Source: CAD feature listing. Evaluate the final solid. Frame: model axes, mm. Give positions to 0.01 mm unless a question says otherwise; leave off trailing zeros. Write each loop counter-clockwise with the first axis right and the second up, starting at its lowest first coordinate (ties: lowest second). Pieces come first, ordered by that corner, then holes. Notation, with made-up numbers: (14, -32.5) -> (38, -32.5) arc R36 ccw to (38, 5.5) -> close; hole circle Ø7 at (11, -37). An arc over 180 degrees is marked (long way). Use one line per item in the form item = value. Start each with the question number.
(1) Cut plane D-D, the plane x = -76.5. Output: boundary loops of the cut face in (y, z), and give its area (3 significant figures).
(2) Cut plane B-B, the plane x = 28.8. Output: boundary loops of the cut face in (y, z).
(3) Cut plane C-C, the plane y = -30. Output: boundary loops of the cut face in (x, z), and give its area (3 significant figures).
(4) First-contact query: P1, Ø3.5, axis at x = -94, y = -30, coming from the +Z side. Flat tip, straight axial feed; report the tip coordinate or a pass-through.
(5) Cut plane A-A, the plane x = 94. Output: boundary loops of the cut face in (y, z), and give its area (3 significant figures).
(6) Material intervals for line 1 along X through (y, z) = (38, 1); line 2 along Y through (x, z) = (-47, 0.25); line 3 along X through (y, z) = (-60, 2.1), sorted ascending. Write a range as from..to.
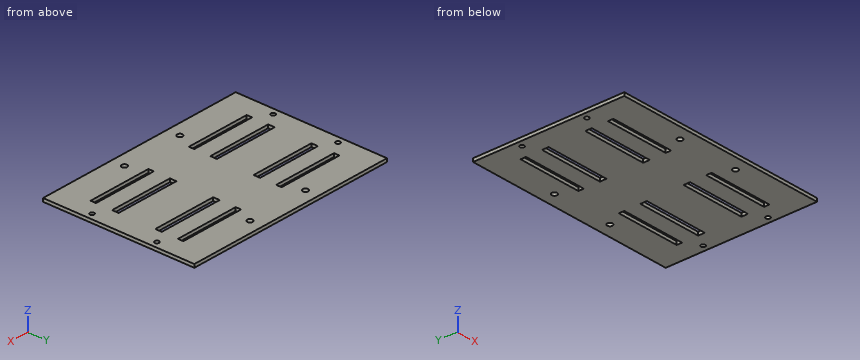
from build123d import *

# Parameters (mm, degrees)
SKETCH_2_W               = 200
SKETCH_2_H               = 140
EXTRUDE_1_DEPTH          = 3
SKETCH_3_R               = 2
CUT_EXTRUDE_1_DEPTH      = 3
SKETCH_4_W               = 60
SKETCH_4_H               = 6
CUT_EXTRUDE_2_DEPTH      = 10
SKETCH_5_W               = 60
SKETCH_5_H               = 5
CUT_EXTRUDE_3_DEPTH      = 6
MIRROR_2_COPY_1_SKETCH_W = 60
MIRROR_2_COPY_1_SKETCH_H = 5
MIRROR_2_COPY_1_DEPTH    = 6
SKETCH_6_R               = 2.5
CUT_EXTRUDE_4_DEPTH      = 5


with BuildPart() as part:
    # 草图2 → 凸台-拉伸1 (new body)
    with BuildSketch(Plane.XY):
        Rectangle(SKETCH_2_W, SKETCH_2_H)
    extrude(amount=EXTRUDE_1_DEPTH)

    # 草图3 → 切除-拉伸1 (cut)
    with BuildSketch(Plane.XY.offset(3)):
        with Locations((94, 30)):
            Circle(SKETCH_3_R)
        with Locations((94, -30)):
            Circle(SKETCH_3_R)
    cut_extrude_1 = extrude(amount=-CUT_EXTRUDE_1_DEPTH, mode=Mode.SUBTRACT)

    # 草图4 → 切除-拉伸2 (cut)
    with BuildSketch(Plane.XY.offset(3)):
        with Locations((51, 20)):
            Rectangle(SKETCH_4_W, SKETCH_4_H)
        with Locations((51, -20)):
            Rectangle(SKETCH_4_W, SKETCH_4_H)
    cut_extrude_2 = extrude(amount=-CUT_EXTRUDE_2_DEPTH, mode=Mode.SUBTRACT)

    # 草图5 → 切除-拉伸3 (cut)
    with BuildSketch(Plane(origin=(0, 0, 0), x_dir=(-1, 0, 0), z_dir=(0, 0, -1))):
        with Locations((-51, 40.40876744)):
            Rectangle(SKETCH_5_W, SKETCH_5_H)
    cut_extrude_3 = extrude(amount=-CUT_EXTRUDE_3_DEPTH, mode=Mode.SUBTRACT)

    # 镜向1: 切除-拉伸3 across plane
    add(cut_extrude_3.mirror(Plane.ZX), mode=Mode.SUBTRACT)

    # 镜向2: 切除-拉伸1, 切除-拉伸2, 切除-拉伸3 across plane
    add(cut_extrude_1.mirror(Plane.ZY), mode=Mode.SUBTRACT)
    add(cut_extrude_2.mirror(Plane.ZY), mode=Mode.SUBTRACT)
    add(cut_extrude_3.mirror(Plane.ZY), mode=Mode.SUBTRACT)

    # 镜向2 copy 1 sketch → 镜向2 copy 1 (cut)
    with BuildSketch(Plane(origin=(0, 0, 0), x_dir=(1, 0, 0), z_dir=(0, 0, -1))):
        with Locations((-51, 40.40876744)):
            Rectangle(MIRROR_2_COPY_1_SKETCH_W, MIRROR_2_COPY_1_SKETCH_H)
    extrude(amount=-MIRROR_2_COPY_1_DEPTH, mode=Mode.SUBTRACT)

    # 草图6 → 切除-拉伸4 (cut)
    with BuildSketch(Plane.XY.offset(3)):
        with Locations((-28.8, 58.108563741)):
            Circle(SKETCH_6_R)
        with Locations((-28.8, -58.108563741)):
            Circle(SKETCH_6_R)
        with Locations((28.8, -58.108563741)):
            Circle(SKETCH_6_R)
        with Locations((28.8, 58.108563741)):
            Circle(SKETCH_6_R)
    extrude(amount=-CUT_EXTRUDE_4_DEPTH, mode=Mode.SUBTRACT)


solid = part.part
Geometry says:
q1.outline = (-70, 0) -> (-42.91, 0) -> (-42.91, 3) -> (-70, 3) -> close; (-37.91, 0) -> (-23, 0) -> (-23, 3) -> (-37.91, 3) -> close; (-17, 0) -> (17, 0) -> (17, 3) -> (-17, 3) -> close; (23, 0) -> (37.91, 0) -> (37.91, 3) -> (23, 3) -> close; (42.91, 0) -> (70, 0) -> (70, 3) -> (42.91, 3) -> close
q1.area = 354 mm^2
q2.outline = (-70, 0) -> (-60.61, 0) -> (-60.61, 3) -> (-70, 3) -> close; (-55.61, 0) -> (-42.91, 0) -> (-42.91, 3) -> (-55.61, 3) -> close; (-37.91, 0) -> (-23, 0) -> (-23, 3) -> (-37.91, 3) -> close; (-17, 0) -> (17, 0) -> (17, 3) -> (-17, 3) -> close; (23, 0) -> (37.91, 0) -> (37.91, 3) -> (23, 3) -> close; (42.91, 0) -> (55.61, 0) -> (55.61, 3) -> (42.91, 3) -> close; (60.61, 0) -> (70, 0) -> (70, 3) -> (60.61, 3) -> close
q3.outline = (-100, 0) -> (-96, 0) -> (-96, 3) -> (-100, 3) -> close; (-92, 0) -> (92, 0) -> (92, 3) -> (-92, 3) -> close; (96, 0) -> (100, 0) -> (100, 3) -> (96, 3) -> close
q3.area = 576 mm^2
q4.P1 = through
q5.outline = (-70, 0) -> (-32, 0) -> (-32, 3) -> (-70, 3) -> close; (-28, 0) -> (28, 0) -> (28, 3) -> (-28, 3) -> close; (32, 0) -> (70, 0) -> (70, 3) -> (32, 3) -> close
q5.area = 396 mm^2
q6.line_1 = -100..-81, -21..21, 81..100
q6.line_2 = -70..-42.91, -37.91..-23, -17..17, 23..37.91, 42.91..70
q6.line_3 = -100..-30.43, -27.17..27.17, 30.43..100
